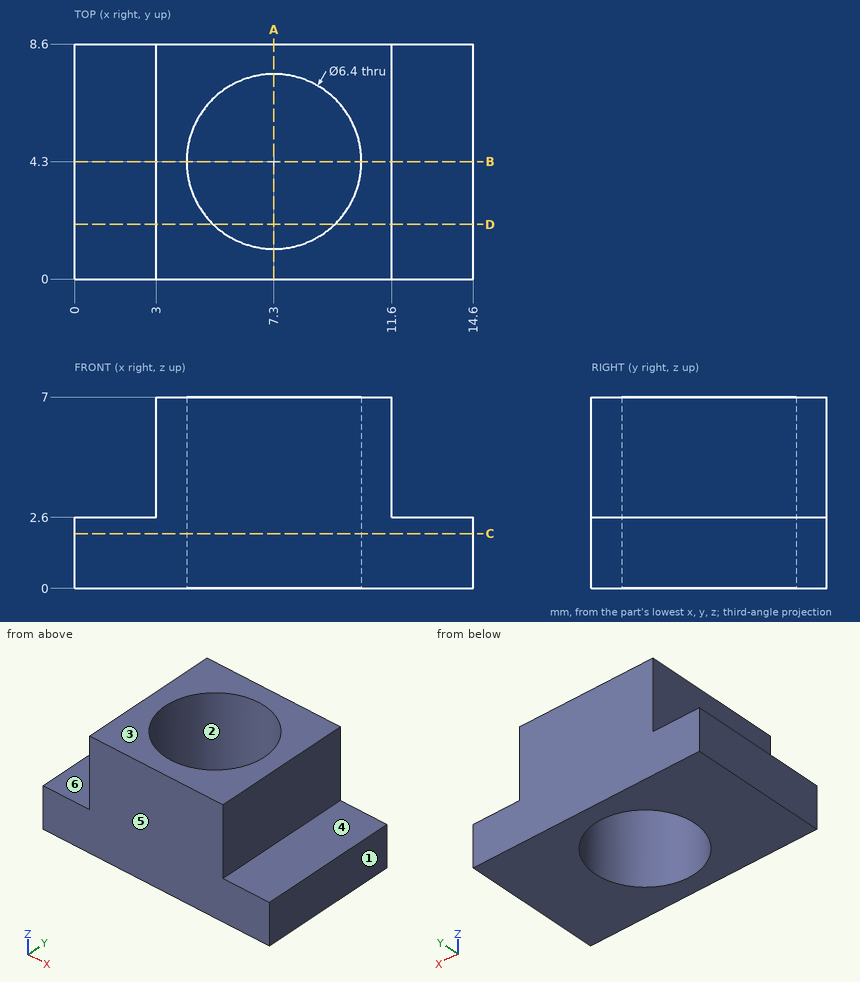
For this review, use the dimensioned drawing (mm, ordinates from the lowest corner) and the shaded views. A direction names the side the tool comes from. Give positions to 0.01 mm unless a question says otherwise; leave off trailing zeros. Write each loop counter-clockwise with the first axis right and the second up, starting at its lowest first coordinate (ties: lowest second). Pieces come first, ordered by that corner, then holes. Notation, with made-up numbers: M 89,62 L 108,62 A28 ccw 108,81 Z; hole C -1.75,10 d6. An arc over 180 degrees is marked long. Answer as a JSON object with one key per item and string values. Group by question number.
Item 1: Consider section C-C on z = 2. Write out the cut boundary in (x, y), plus the area to 3 significant figures.
Item 2: For probe 1 along Y at (x, z) = (7.3, 4.5); probe 2 along Z at (x, y) = (13.5, 5.25); probe 3 along Y at (x, z) = (6.5, 3.5), list the stretches that pass through material, from the lowest coordinate up. Write a range as [from, to].
Item 3: Consider section D-D on y = 2. Write out the cut boundary in (x, z).
Item 4: Tool access review of the marked faces 4, 5 and 6: name each direction out of +Z, -Z, +X, -X, +Y, -Y from which nothing blocks a thin tool from reaching the whole face with its end or side.
Item 5: For pin 1 Ø0.9 at (x, y) = (2, 6) entering from +Z; pin 2 Ø3.5 at (y, z) = (5, 6) entering from -X, all flat-tipped, find the tip position at first contact; note any pin that passes through.
Item 6: Consider section A-A on x = 7.3. Write out the cut boundary in (y, z), plus the area to 3 significant figures.
Item 7: Draft analysis for pull direction X (two halves, no side actions). For the marked faces 1, 2 and 3, state which applies: +X half, -X half, draft (parallel to the pull), parting line (faces both ways), or undercut.
Item 8: Consider section B-B on y = 4.3. Write out the cut boundary in (x, z), plus the area to 3 significant figures.
Check result:
{
 "1": {"outline": "M 0,0 L 14.6,0 L 14.6,8.6 L 0,8.6 Z; hole C 7.3,4.3 d6.4", "area": "93.4 mm^2"},
 "2": {"probe 1": "y = [0, 1.1], [7.5, 8.6]", "probe 2": "z = [0, 2.6]", "probe 3": "y = [0, 1.2], [7.4, 8.6]"},
 "3": {"outline": "M 0,0 L 5.08,0 L 5.08,7 L 3,7 L 3,2.6 L 0,2.6 Z; M 9.52,0 L 14.6,0 L 14.6,2.6 L 11.6,2.6 L 11.6,7 L 9.52,7 Z"},
 "4": {"face 4": "+Z, +X, +Y, -Y", "face 5": "+Z, -Z, +X, -X, -Y", "face 6": "+Z, -X, +Y, -Y"},
 "5": {"pin 1": "stops at z = 2.6", "pin 2": "stops at x = 3"},
 "6": {"outline": "M 0,0 L 1.1,0 L 1.1,7 L 0,7 Z; M 7.5,0 L 8.6,0 L 8.6,7 L 7.5,7 Z", "area": "15.4 mm^2"},
 "7": {"face 1": "+X half", "face 2": "undercut", "face 3": "draft"},
 "8": {"outline": "M 0,0 L 4.1,0 L 4.1,7 L 3,7 L 3,2.6 L 0,2.6 Z; M 10.5,0 L 14.6,0 L 14.6,2.6 L 11.6,2.6 L 11.6,7 L 10.5,7 Z", "area": "31.0 mm^2"}
}
